from build123d import *

# Parameters (mm, degrees)
SKETCH1_R           = 2.1
BOSS_EXTRUDE1_DEPTH = 4.5
SKETCH2_R           = 2.2
SKETCH2_W           = 41.1
SKETCH2_H           = 20.5
CUT_EXTRUDE1_DEPTH  = 10
SKETCH3_W           = 100
SKETCH3_H           = 20
CUT_EXTRUDE2_DEPTH  = 10


with BuildPart() as part:
    # Sketch1 → Boss-Extrude1 (new body)
    with BuildSketch(Plane(origin=(0, 0, 0), x_dir=(1, 0, 0), z_dir=(0, 1, 0))):
        Polygon((20, 40), (50, 25), (50, -25), (-50, -25), (-50, 25), (-20, 40), align=None)
        with Locations((-41, 15)):
            Circle(SKETCH1_R, mode=Mode.SUBTRACT)
        with Locations((41, 15)):
            Circle(SKETCH1_R, mode=Mode.SUBTRACT)
        with Locations((-21, 15)):
            Circle(SKETCH1_R, mode=Mode.SUBTRACT)
        with Locations((21, 15)):
            Circle(SKETCH1_R, mode=Mode.SUBTRACT)
    extrude(amount=BOSS_EXTRUDE1_DEPTH)

    # Sketch2 → Cut-Extrude1 (cut)
    with BuildSketch(Plane.XZ):
        with Locations((13.2, -19.9)):
            Circle(SKETCH2_R)
        with Locations((13.2, -10.1)):
            Circle(SKETCH2_R)
        with Locations((-35.2, -19.9)):
            Circle(SKETCH2_R)
        with Locations((-35.2, -10.1)):
            Circle(SKETCH2_R)
        with Locations((-11, -15)):
            Rectangle(SKETCH2_W, SKETCH2_H)
    extrude(amount=-CUT_EXTRUDE1_DEPTH, mode=Mode.SUBTRACT)

    # Sketch3 → Cut-Extrude2 (cut)
    with BuildSketch(Plane.XZ):
        with Locations((0, 15)):
            Rectangle(SKETCH3_W, SKETCH3_H)
    extrude(amount=-CUT_EXTRUDE2_DEPTH, mode=Mode.SUBTRACT)


solid = part.part
Verification items for the finished model (mm, model axes). A direction names the side the tool comes from. Give positions to 0.01 mm unless a question says otherwise; leave off trailing zeros. Loops run counter-clockwise (first coordinate to the right, second up) from the corner with the lowest first, then second, coordinate; pieces in that order, holes last.
1) Depth check by flat-ended pin: pin 1 Ø4 at (x, z) = (41, -15) entering from -Y; pin 2 Ø1 at (y, z) = (3, -30) entering from -X; pin 3 Ø1.5 at (x, y) = (-39.5, 4) entering from -Z (3 decimals). Enter the tip coordinate at first touch or a pass-through.
2) Sectioned sample at A-A, the plane x = -41. Enter the section's corners in (y, z), then the cut area to 3 significant figures.
3) Thickness scan on line 1 along Z through (x, y) = (13.2, 2.9); line 2 along X through (y, z) = (3.6, -10); line 3 along X through (y, z) = (1.9, -15). Record the ranges inside material, lowest first.
4) Draft check along X on faces 1 (the flat face through (50, 2, -10)), 2 (the cylindrical face through (12.91, 2.22, -17.72)), 3 (the flat face through (11.8, 0, -17.8)). Enter one of: pulls with the +X half, pulls with the -X half, needs draft (parallel to the pull), parting line crosses it, or undercut.
5) Sectioned sample at B-B, the plane z = -19.9. Enter the section's corners in (x, y), then the cut area to 3 significant figures.
6) Set-up check for faces 4 (the flat face through (0, 2, -40)), 5 (the flat face through (-11, 2, -25.25)): record each of +Z, -Z, +X, -X, +Y, -Y from which the full face is reachable in a straight line by a thin tool's end or side.
7) Sectioned sample at D-D, the plane y = 1.2. Count the separate pieces of the cut face and the enclosed holes in it, then the cut area to 3 significant figures.
8) Sectioned sample at C-C, the plane x = 13.2. Enter the section's corners in (y, z).
Answers:
1. pin 1: passes through
1. pin 2: stops at x = -41
1. pin 3: stops at z = -30.625
2. outline: (0, -29.5) - (4.5, -29.5) - (4.5, -17.1) - (0, -17.1) - close; (0, -12.9) - (4.5, -12.9) - (4.5, 5) - (0, 5) - close
2. area: 136 mm2
3. line 1: z = -40 to -22.1, -17.7 to -12.3, -7.9 to 5
3. line 2: x = -50 to -37.4, -33 to -31.55, 9.55 to 11, 15.4 to 50
3. line 3: x = -50 to -43.1, -38.9 to -31.55, 9.55 to 18.9, 23.1 to 38.9, 43.1 to 50
4. face 1: pulls with the +X half
4. face 2: undercut
4. face 3: needs draft
5. outline: (-50, 0) - (-37.4, 0) - (-37.4, 4.5) - (-50, 4.5) - close; (-33, 0) - (-31.55, 0) - (-31.55, 4.5) - (-33, 4.5) - close; (9.55, 0) - (11, 0) - (11, 4.5) - (9.55, 4.5) - close; (15.4, 0) - (50, 0) - (50, 4.5) - (15.4, 4.5) - close
5. area: 225 mm2
6. face 4: -Z, +X, -X, +Y, -Y
6. face 5: +Y, -Y
7. separate pieces: 1
7. enclosed holes: 8
7. area: 3,110 mm2
8. outline: (0, -40) - (4.5, -40) - (4.5, -22.1) - (0, -22.1) - close; (0, -17.7) - (4.5, -17.7) - (4.5, -12.3) - (0, -12.3) - close; (0, -7.9) - (4.5, -7.9) - (4.5, 5) - (0, 5) - close
